Read the model definition and answer for the solid it produces. Units are mm, in the model's axes. A direction names the side the tool comes from. Coordinates: 2 decimals unless noted, no trailing zeros. Write each loop counter-clockwise with the first axis right and the second up, starting at its lowest first coordinate (ties: lowest second). Pieces come first, ordered by that corner, then holes. Notation, with made-up numbers: (77, 16.5) -> (98, 16.5) arc R23 ccw to (98, 41.5) -> close; hole circle Ø9 at (82, -7). An arc over 180 degrees is marked (long way). Use CSV: the item, a comma, the result in double quotes.
from build123d import *

# Parameters (mm, degrees)
SKIZZE1_W                         = 4.5
SKIZZE1_H                         = 11.423295
AUFSATZ_LINEAR_AUSTRAGEN1_DEPTH   = 4.5
SKIZZE1_W_2                       = 4.451373
AUFSATZ_LINEAR_AUSTRAGEN1_2_DEPTH = 4.5
SKIZZE2_R                         = 2.5
AUFSATZ_LINEAR_AUSTRAGEN2_DEPTH   = 10
VERRUNDUNG4_R                     = 1


with BuildPart() as part:
    # Skizze1 → Aufsatz-Linear austragen1 (new body)
    with BuildSketch(Plane.XY):
        with Locations((-2.25, 5.7116475)):
            Rectangle(SKIZZE1_W, SKIZZE1_H)
    extrude(amount=AUFSATZ_LINEAR_AUSTRAGEN1_DEPTH)



with BuildPart() as body_2:
    # Skizze1 → Aufsatz-Linear austragen1 2 (new body)
    with BuildSketch(Plane.XY):
        with Locations((12.2256865, 5.7116475)):
            Rectangle(SKIZZE1_W_2, SKIZZE1_H)
    extrude(amount=AUFSATZ_LINEAR_AUSTRAGEN1_2_DEPTH)


with BuildPart() as part_1:
    add(part.part)

    add(body_2.part)  # Aufsatz-Linear austragen2 merges body 2
    # Skizze2 → Aufsatz-Linear austragen2 (add)
    with BuildSketch(Plane(origin=(0, 0, 0), x_dir=(0, 0, -1), z_dir=(1, 0, 0))):
        with Locations(Location((-2.520313205, 9.586549386, 0), (0, 0, 217.638946457))):
            Circle(SKIZZE2_R)
    extrude(amount=AUFSATZ_LINEAR_AUSTRAGEN2_DEPTH)

    # Verrundung4
    # the kernel refuses this fillet: 1 mm, written as the material it takes off along each edge
    with BuildSketch(Plane(origin=(16.951373, 11.423295, 0), x_dir=(0, 0, 1), z_dir=(-1, 0, 0)), Plane(origin=(16.951373, 11.423295, 4.5), x_dir=(0, -1, 0), z_dir=(-1, 0, 0))) as verrundung4_piece_1:
        with BuildLine():
            CenterArc((VERRUNDUNG4_R, -VERRUNDUNG4_R), VERRUNDUNG4_R, 90, 90)
            Line((0, -VERRUNDUNG4_R), (0, 0))
            Line((0, 0), (VERRUNDUNG4_R, 0))
        make_face()
    extrude(amount=6.951373, mode=Mode.SUBTRACT)
    with BuildSketch(Plane(origin=(14.451373, 11.423295, -2.5), x_dir=(-1, 0, 0), z_dir=(0, 0, 1)), Plane(origin=(-4.5, 11.423295, -2.5), x_dir=(0, -1, 0), z_dir=(0, 0, 1))) as verrundung4_piece_2:
        with BuildLine():
            CenterArc((VERRUNDUNG4_R, VERRUNDUNG4_R), VERRUNDUNG4_R, 180, 90)
            Line((0, VERRUNDUNG4_R), (0, 0))
            Line((0, 0), (VERRUNDUNG4_R, 0))
        make_face()
    extrude(amount=9.5, mode=Mode.SUBTRACT)
    with BuildSketch(Plane(origin=(-7, 11.423295, 0), x_dir=(0, -1, 0), z_dir=(1, 0, 0))) as verrundung4_piece_3:
        with BuildLine():
            CenterArc((VERRUNDUNG4_R, -VERRUNDUNG4_R), VERRUNDUNG4_R, 90, 90)
            Line((0, -VERRUNDUNG4_R), (0, 0))
            Line((0, 0), (VERRUNDUNG4_R, 0))
        make_face()
    extrude(amount=7, mode=Mode.SUBTRACT)
    with BuildSketch(Plane(origin=(-7, 11.423295, 4.5), x_dir=(0, -1, 0), z_dir=(1, 0, 0))) as verrundung4_piece_4:
        with BuildLine():
            CenterArc((VERRUNDUNG4_R, VERRUNDUNG4_R), VERRUNDUNG4_R, 180, 90)
            Line((0, VERRUNDUNG4_R), (0, 0))
            Line((0, 0), (VERRUNDUNG4_R, 0))
        make_face()
    extrude(amount=7, mode=Mode.SUBTRACT)


solid = part_1.part
1. A cutting plane is placed at C-C (z = 2.7). Give the vertices of the cut face in (x, y).
Solutions:
outline,"(-4.5, 0) -> (0, 0) -> (0, 7.09) -> (10, 7.09) -> (10, 0) -> (14.45, 0) -> (14.45, 10.42) arc R1 ccw to (13.45, 11.42) -> (10, 11.42) -> (10, 12.08) -> (0, 12.08) -> (0, 11.42) -> (-3.5, 11.42) arc R1 ccw to (-4.5, 10.42) -> close"
2. Each of these flat-tipped pins is pushed along its axis until it touches: pin 1 Ø3 at (x, y) = (4.5, 6) entering from -Z; pin 2 Ø3 at (x, y) = (3.5, 6.5) entering from -Z; pin 3 Ø2 at (x, y) = (2.5, 2) entering from -Z; pin 4 Ø1.3 at (x, y) = (-2, 3) entering from +Z. Where does it stop, or does it pass through?
Solutions:
pin 1,"stops at z = 1.14"
pin 2,"stops at z = 0.59"
pin 3,"passes through"
pin 4,"stops at z = 4.5"
3. A tool of negligible diameter and unlimited length cuts with its end or side. For faces 1 (the flat face through (12, 11.423, 2)), 2 (the cylindrical face through (12.257, 11.123, 4.215)), 3 (the cylindrical face through (-2.28, 11.14, 4.2)), from which of +Z, -Z, +X, -X, +Y, -Y can it reach the whole face along a straight path? Write none if from no direction.
Solutions:
face 1,"+Z, -Z, +X, +Y"
face 2,"+Z, +X, +Y"
face 3,"+Z, -X, +Y"
4. A cutting plane is placed at D-D (y = 8.75). Give the vertices of the cut face in (x, z).
Solutions:
outline,"(-4.5, 0) -> (0, 0) -> (0, 0.16) -> (10, 0.16) -> (10, 0) -> (14.45, 0) -> (14.45, 4.5) -> (10, 4.5) -> (10, 4.88) -> (0, 4.88) -> (0, 4.5) -> (-4.5, 4.5) -> close"
5. A cutting plane is placed at B-B (x = 11). Give the vertices of the cut face in (y, z).
Solutions:
outline,"(0, 0) -> (10.42, 0) arc R1 ccw to (11.42, 1) -> (11.42, 3.5) arc R1 ccw to (10.42, 4.5) -> (0, 4.5) -> close"
6. For a pull along X with two mould halves and no side action, classify faces 4 (the flat face through (10, 11.6, 3.6)), 5 (the flat face through (-2, 0, 2)), 6 (the flat face through (0, 4, 2)), 7 (the cylindrical face through (-4.2, 11.14, 2.22)) as pulls with the +X half, pulls with the -X half, needs draft (parallel to the pull), parting line crosses it, or undercut.
Solutions:
face 4,"pulls with the +X half"
face 5,"needs draft"
face 6,"undercut"
face 7,"pulls with the -X half"
7. A cutting plane is placed at A-A (y = 2.5). Give the vertices of the cut face in (x, z), and give its area (3 significant figures).
Solutions:
outline,"(-4.5, 0) -> (0, 0) -> (0, 4.5) -> (-4.5, 4.5) -> close; (10, 0) -> (14.45, 0) -> (14.45, 4.5) -> (10, 4.5) -> close"
area,"40.3 mm^2"
8. Find the intervals of material crossed by line 1 along X through (y, z) = (7.75, 0.35); line 2 along Y through (x, z) = (3.5, 2.6); line 3 along Z through (x, y) = (13.5, 8.75), in increasing order.
Solutions:
line 1,"x = -4.5 to 0, 10 to 14.45"
line 2,"y = 7.09 to 12.09"
line 3,"z = 0 to 4.5"
